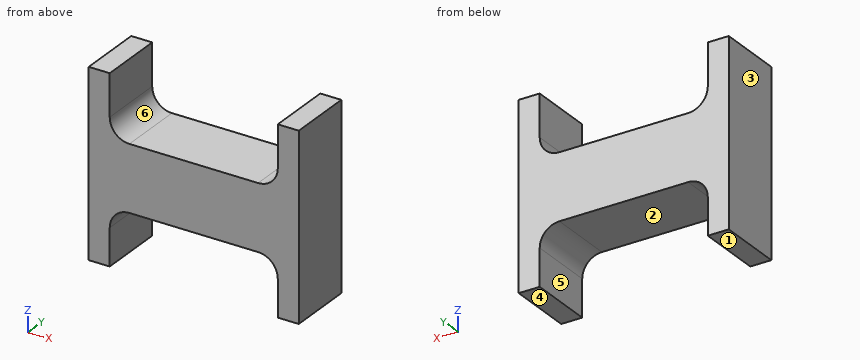
from build123d import *

# Parameters (mm, degrees)
F1_DEPTH = 25


with BuildPart() as f1:
    # F0 (on Front) → F1 (new body)
    with BuildSketch(Plane.XZ):
        with BuildLine():
            Line((-31.33769, 35.93692), (-39.33769, 35.93692))
            Line((-39.33769, 35.93692), (-39.33769, -34.06308))
            Line((-39.33769, -34.06308), (-31.33769, -34.06308))
            Line((-31.33769, -34.06308), (-31.33769, -20))
            ThreePointArc((-31.33769, -20), (-29.140991, -14.696699), (-23.83769, -12.5))
            Line((-23.83769, -12.5), (25.16231, -12.5))
            ThreePointArc((25.16231, -12.5), (30.465611, -14.696699), (32.66231, -20))
            Line((32.66231, -20), (32.66231, -34.06308))
            Line((32.66231, -34.06308), (40.66231, -34.06308))
            Line((40.66231, -34.06308), (40.66231, 35.93692))
            Line((40.66231, 35.93692), (32.66231, 35.93692))
            Line((32.66231, 35.93692), (32.66231, 20))
            ThreePointArc((32.66231, 20), (30.465611, 14.696699), (25.16231, 12.5))
            Line((25.16231, 12.5), (-23.83769, 12.5))
            ThreePointArc((-23.83769, 12.5), (-29.140991, 14.696699), (-31.33769, 20))
            Line((-31.33769, 20), (-31.33769, 35.93692))
        make_face()
    extrude(amount=F1_DEPTH)


solid = f1.part
Design review of the part built by this model. Coordinates are the model's own, in mm. Face numbers are marked on the shaded views. A direction names the side the tool comes from. Round coordinates to 2 decimals unless told otherwise and drop trailing zeros. Write each loop counter-clockwise with the first axis right and the second up, starting at its lowest first coordinate (ties: lowest second). Pieces come first, ordered by that corner, then holes.
Item 1: For the marked faces 4, 5 and 6, list the 3-axis set-ups (+Z, -Z, +X, -X, +Y, -Y) from which the entire face can be reached by the end or side of a thin tool; tool diameter is ignored.
Item 2: Consider section C-C on x = -12. Give the boundary of the cut face in (y, z).
Item 3: Consider section D-D on x = 31.5. Give the boundary of the cut face in (y, z).
Item 4: Consider section B-B on y = -15.5. Give the boundary of the cut face in (x, z), and give its area (3 significant figures).
Item 5: For pin 1 Ø6 at (x, y) = (-2, -22) entering from +Z; pin 2 Ø12.5 at (x, y) = (-4, -14) entering from -Z, all flat-tipped, find the tip position at first contact; note any pin that passes through.
Item 6: Wall thickness on L1, parallel to X at y = -3.25, z = -21; L2, parallel to Z at x = -19.5, y = -13; L3, parallel to X at y = -12, z = -17: over which ranges is each line inside the solid? List them lowest first.
Item 7: Consider section A-A on z = 23.5. Give the boundary of the cut face in (x, y).
Item 8: Draft analysis for pull direction X (two halves, no side actions). For the marked faces 1, 2 and 3, state which applies: released by +X, released by -X, zero draft, split by the parting line, or undercut.
Check values:
1. face 4: -Z, +X, -X, +Y, -Y
1. face 5: -Z, +Y, -Y
1. face 6: +Z, +Y, -Y
2. outline: (-25, -12.5) - (0, -12.5) - (0, 12.5) - (-25, 12.5) - close
3. outline: (-25, -15.99) - (0, -15.99) - (0, 15.99) - (-25, 15.99) - close
4. outline: (-39.34, -34.06) - (-31.34, -34.06) - (-31.34, -20) arc R7.5 cw to (-23.84, -12.5) - (25.16, -12.5) arc R7.5 cw to (32.66, -20) - (32.66, -34.06) - (40.66, -34.06) - (40.66, 35.94) - (32.66, 35.94) - (32.66, 20) arc R7.5 cw to (25.16, 12.5) - (-23.84, 12.5) arc R7.5 cw to (-31.34, 20) - (-31.34, 35.94) - (-39.34, 35.94) - close
4. area: 2,770 mm2
5. pin 1: stops at z = 12.5
5. pin 2: stops at z = -12.5
6. L1: x = -39.34 to -31.34, 32.66 to 40.66
6. L2: z = -12.5 to 12.5
6. L3: x = -39.34 to -30.71, 32.04 to 40.66
7. outline: (-39.34, -25) - (-31.34, -25) - (-31.34, 0) - (-39.34, 0) - close; (32.66, -25) - (40.66, -25) - (40.66, 0) - (32.66, 0) - close
8. face 1: zero draft
8. face 2: undercut
8. face 3: released by -X
